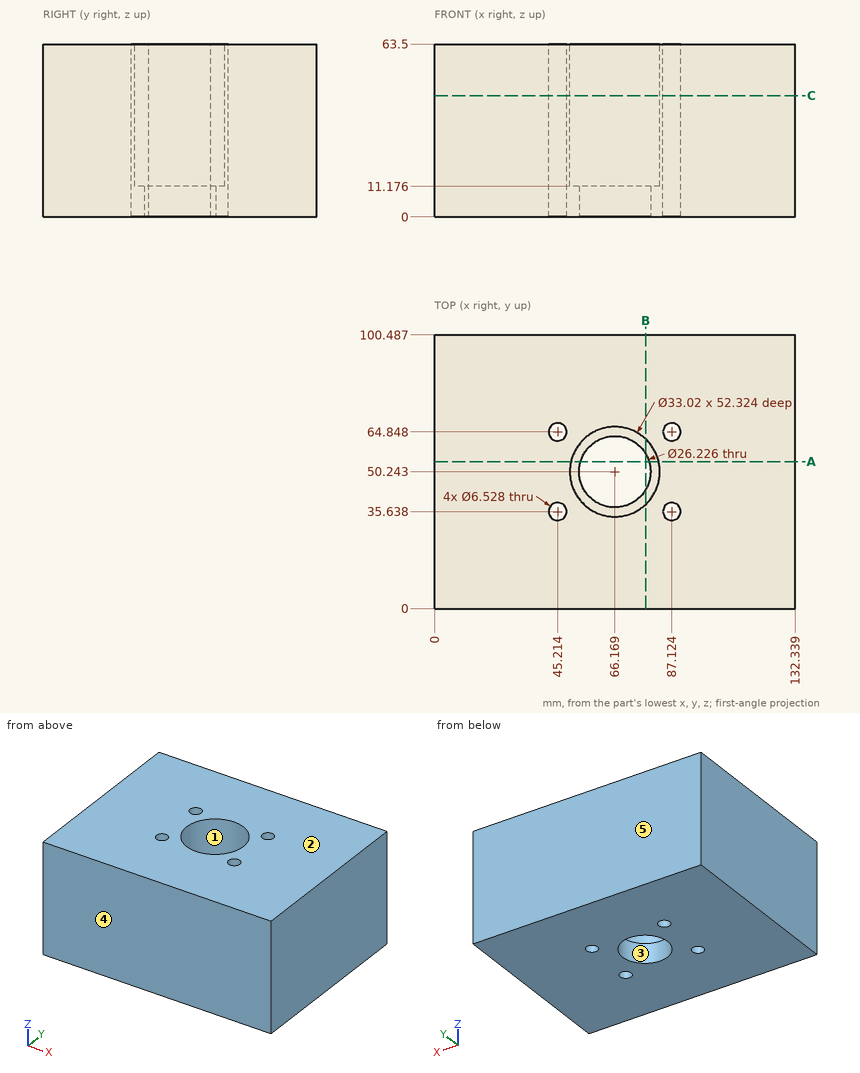
Verification items for this drawing (mm, ordinates from the low corner). A direction names the side the tool comes from. Coordinates: 2 decimals unless noted, no trailing zeros. Write each loop counter-clockwise with the first axis right and the second up, starting at its lowest first coordinate (ties: lowest second). Pieces come first, ordered by that corner, then holes. Notation, with made-up numbers: (-32.75, -21.75) -> (21.25, -21.75) arc R5 cw to (21.25, -14.75) -> close; hole circle Ø5 at (79.25, 62.25). An arc over 180 degrees is marked (long way). One line per item, written item: value. Start each with the question number.
Q1. Mould release check, pull along Y, two halves, no side actions. Record for the marked faces 3, 4 and 5: pulls with the +Y half, pulls with the -Y half, needs draft (parallel to the pull), parting line crosses it, or undercut.
Q2. Access from +Z, -Z, +X, -X, +Y, -Y to the whole of each face (thin tool, end or side, straight path). Record for the marked faces 1 and 2.
Q3. Cross-section at A-A on y = 54. Enter the section's corners in (x, z) (1 decimal), and give its area (3 significant figures).
Q4. Cross-section at C-C on z = 44.5. State how many separate pieces and enclosed holes the cut face has, and give its area (3 significant figures).
Q5. Go/stop test with a flat-tipped pin: P1, Ø6, axis at x = 45.21, y = 35.64, coming from the -Z side. Record where the tip stops, or that it passes through.
Q6. Cross-section at B-B on x = 77.5. Enter the section's corners in (y, z) (1 decimal), and give its area (3 significant figures).
Q7. Thickness scan on L1, parallel to X at y = 36, z = 37.5 (1 decimal); L2, parallel to Y at x = 58.5, z = 5.5 (1 decimal); L3, parallel to Z at x = 63, y = 35.5 (1 decimal). Record the ranges inside material, lowest first. Write a range as from..to.
Checked values:
1. face 3: undercut
1. face 4: pulls with the -Y half
1. face 5: pulls with the +Y half
2. face 1: +Z
2. face 2: +Z, +X, -X, +Y, -Y
3. outline: (0, 0) -> (53.6, 0) -> (53.6, 11.2) -> (50.1, 11.2) -> (50.1, 63.5) -> (0, 63.5) -> close; (78.7, 0) -> (132.3, 0) -> (132.3, 63.5) -> (82.2, 63.5) -> (82.2, 11.2) -> (78.7, 11.2) -> close
3. area: 6,440 mm²
4. separate pieces: 1
4. enclosed holes: 5
4. area: 12,300 mm²
5. P1: passes through
6. outline: (0, 0) -> (43.6, 0) -> (43.6, 11.2) -> (38.2, 11.2) -> (38.2, 63.5) -> (0, 63.5) -> close; (56.8, 0) -> (100.5, 0) -> (100.5, 63.5) -> (62.3, 63.5) -> (62.3, 11.2) -> (56.8, 11.2) -> close
6. area: 4,980 mm²
7. L1: x = 0..42, 48.5..57.8, 74.5..83.9, 90.4..132.3
7. L2: y = 0..39.6, 60.9..100.5
7. L3: z = 0..11.2
